Could you check a few things on this model? Use its own coordinates, in mm. A direction names the side the tool comes from. Round coordinates to 2 decimals unless told otherwise and drop trailing zeros. Loops run counter-clockwise (first coordinate to the right, second up) from the corner with the lowest first, then second, coordinate; pieces in that order, holes last. Notation, with made-up numbers: (59.25, -17) -> (66.25, -17) arc R32 cw to (66.25, 15) -> close; hole circle Ø11 at (-37.5, 3.25). An arc over 180 degrees is marked (long way). Write each question's results on one line, items separated by ' | '. Start each with the question number.
1) Which directions (+Z, -Z, +X, -X, +Y, -Y) give clear straight access to the entire face, cutting with the end or side of a thin tool? Please do faces 5 (the flat face through (68, 108.931, 6)), 6 (the cylindrical face through (65.776, 3.849, 6.439)), 7 (the flat face through (91.251, 120, 6)), 8 (the flat face through (107, 0, 6)), 9 (the flat face through (73, 98.39, 6)).
2) If I drill on probe 1 along X at (y, z) = (108, 5.25); probe 2 along X at (y, z) = (112, 6.25); probe 3 along Y at (x, z) = (108, 9.5), over which ranges is the centre line in solid material (lowest first)?
3) For P1, Ø5.5, axis at x = 142, z = 4.5, coming from the +Y side; P2, Ø4, axis at x = 127.5, z = 6.5, coming from the +Y side; P3, Ø0.7, axis at x = 146.5, z = 7.5, coming from the -Y side; P4, Ø20, axis at x = 107.13, y = 38.63, coming from the -Z side, each with a flat end and sliding along its axis, tell me the tip position at first contact or that it passes through.
4) We'd pull the mould along X, two halves only. Please class faces 1 (the flat face through (62.126, 63, 6)), 2 (the flat face through (75.868, 101, 6)), 3 (the flat face through (147.35, 106, 6)), 4 (the cylindrical face through (148.277, 3.65, 6.439)): pulls with the +X half, pulls with the -X half, needs draft (parallel to the pull), parting line crosses it, or undercut.
5) Imagine slicing it at A-A, the plane x = 102. List the corners of the cut face in (y, z) for me.
6) Imagine slicing it at C-C, the plane x = 117.5. List the corners of the cut face in (y, z) for me, plus the area to 3 significant figures.
7) Imagine slicing it at B-B, the plane x = 86. List the corners of the cut face in (y, z) for me.
from build123d import *

# Parameters (mm, degrees)
SKETCH12_W           = 90
SKETCH12_H           = 113.63
BOSS_EXTRUDE10_DEPTH = 12.7
SKETCH25_R           = 18.5
CUT_EXTRUDE1_DEPTH   = 191.303286742
SKETCH26_R           = 18.5
SKETCH26_R_2         = 16.5
BOSS_EXTRUDE15_DEPTH = 5.7
FILLET1_R            = 12.8
CUT_EXTRUDE2_DEPTH   = 191.303286742
BOSS_EXTRUDE16_DEPTH = 12.7


with BuildPart() as part:
    # Sketch12 → Boss-Extrude10 (new body)
    with BuildSketch(Plane.XY):
        with Locations((107.125849364, 56.815)):
            Rectangle(SKETCH12_W, SKETCH12_H)
    extrude(amount=BOSS_EXTRUDE10_DEPTH)

    # Sketch25 → Cut-Extrude1 (cut, through all)
    with BuildSketch(Plane.XY.offset(12.7)):
        with Locations((107.125849364, 38.627603634)):
            Circle(SKETCH25_R)
    extrude(amount=-CUT_EXTRUDE1_DEPTH, mode=Mode.SUBTRACT)

    # Sketch26 → Boss-Extrude15 (add)
    with BuildSketch(Plane.XY.offset(12.7)):
        with Locations((107.125849364, 38.627603634)):
            Circle(SKETCH26_R)
        with Locations((107.125849364, 38.627603634)):
            Circle(SKETCH26_R_2, mode=Mode.SUBTRACT)
    extrude(amount=-BOSS_EXTRUDE15_DEPTH)

    # Fillet1
    fillet1_edges = [part.edges().sort_by_distance(p)[0] for p in [
        (62.125849364, 0, 6.35),
        (152.125849364, 0, 6.35),
    ]]
    fillet(fillet1_edges, radius=FILLET1_R)

    # Sketch27 → Cut-Extrude2 (cut, through all)
    with BuildSketch(Plane(origin=(0, 0, 0), x_dir=(-1, 0, 0), z_dir=(0, 0, -1))):
        Polygon((-69.263849364, 108.931), (-69.263849364, 113.63), (-75.867849364, 113.63), (-75.867849364, 108.931), (-78.229849364, 108.931), (-78.229849364, 103.089), (-75.867849364, 103.089), (-75.867849364, 98.39), (-69.263849364, 98.39), (-69.263849364, 103.089), (-66.901849364, 103.089), (-66.901849364, 108.931), align=None)
        Polygon((-138.383849364, 108.931), (-138.383849364, 113.63), (-144.987849364, 113.63), (-144.987849364, 108.931), (-147.349849364, 108.931), (-147.349849364, 103.089), (-144.987849364, 103.089), (-144.987849364, 98.39), (-138.383849364, 98.39), (-138.383849364, 103.089), (-136.021849364, 103.089), (-136.021849364, 108.931), align=None)
    extrude(amount=-CUT_EXTRUDE2_DEPTH, mode=Mode.SUBTRACT)

    # Sketch28 → Boss-Extrude16 (add)
    with BuildSketch(Plane(origin=(0, 113.63, 0), x_dir=(1, 0, 0), z_dir=(0, 1, 0))):
        Polygon((107.125849364, 0), (91.250849364, 0), (91.250849364, -12.7), (123.000849364, -12.7), (123.000849364, 0), align=None)
    extrude(amount=BOSS_EXTRUDE16_DEPTH)


solid = part.part
Checked values:
1) face 5: +Z, -Z | face 6: +Z, -Z, -X, -Y | face 7: +Z, -Z, -X, +Y | face 8: +Z, -Z, +X, -X, -Y | face 9: +Z, -Z, +Y
2) probe 1: 62.13 to 66.9, 78.23 to 136.02, 147.35 to 152.13 | probe 2: 62.13 to 69.26, 75.87 to 138.38, 144.99 to 152.13 | probe 3: 0 to 22.15, 55.1 to 126.33
3) P1: y = 98.39 | P2: y = 113.63 | P3: y = 1.97 | P4: through
4) face 1: pulls with the -X half | face 2: undercut | face 3: undercut | face 4: pulls with the +X half
5) outline: (0, 0) -> (20.85, 0) -> (20.85, 7) -> (22.94, 7) -> (22.94, 12.7) -> (0, 12.7) -> close; (54.31, 7) -> (56.4, 7) -> (56.4, 0) -> (126.33, 0) -> (126.33, 12.7) -> (54.31, 12.7) -> close
6) outline: (0, 0) -> (23.31, 0) -> (23.31, 7) -> (25.8, 7) -> (25.8, 12.7) -> (0, 12.7) -> close; (51.46, 7) -> (53.95, 7) -> (53.95, 0) -> (126.33, 0) -> (126.33, 12.7) -> (51.46, 12.7) -> close | area: 1,240 mm^2
7) outline: (0, 0) -> (113.63, 0) -> (113.63, 12.7) -> (0, 12.7) -> close
